Source: CAD feature listing. Evaluate the final solid. Frame: model axes, mm. A direction names the side the tool comes from. Round coordinates to 2 decimals unless told otherwise and drop trailing zeros. Write each loop counter-clockwise with the first axis right and the second up, starting at its lowest first coordinate (ties: lowest second). Pieces come first, ordered by that corner, then holes.
```python
from build123d import *

# Parameters (mm, degrees)
SKETCH1_W           = 15
SKETCH1_H           = 25.4
BOSS_EXTRUDE1_DEPTH = 3.175
SKETCH2_W           = 15
SKETCH2_H           = 3.175
BOSS_EXTRUDE2_DEPTH = 22.225
SKETCH3_R           = 1.5
CUT_EXTRUDE2_DEPTH  = 39.927111375
SKETCH4_R           = 1.5
CUT_EXTRUDE3_DEPTH  = 37.933868265


with BuildPart() as part:
    # Sketch1 → Boss-Extrude1 (new body)
    with BuildSketch(Plane(origin=(0, 0, 0), x_dir=(0, 0, -1), z_dir=(1, 0, 0))):
        with Locations((7.5, 12.7)):
            Rectangle(SKETCH1_W, SKETCH1_H)
    extrude(amount=BOSS_EXTRUDE1_DEPTH)

    # Sketch2 → Boss-Extrude2 (add)
    with BuildSketch(Plane(origin=(3.175, 0, 0), x_dir=(0, 0, -1), z_dir=(1, 0, 0))):
        with Locations((7.5, 1.5875)):
            Rectangle(SKETCH2_W, SKETCH2_H)
    extrude(amount=BOSS_EXTRUDE2_DEPTH)

    # Sketch3 → Cut-Extrude2 (cut, through all)
    with BuildSketch(Plane.XZ):
        with Locations(Location((7.5, -7.5, 0), (0, 0, 270))):
            Circle(SKETCH3_R)
        with Locations(Location((15, -7.5, 0), (0, 0, 270))):
            Circle(SKETCH3_R)
    extrude(amount=-CUT_EXTRUDE2_DEPTH, mode=Mode.SUBTRACT)

    # Sketch4 → Cut-Extrude3 (cut, through all)
    with BuildSketch(Plane(origin=(3.175, 0, 0), x_dir=(0, 0, -1), z_dir=(1, 0, 0))):
        with Locations((7.5, 17.9)):
            Circle(SKETCH4_R)
        with Locations((7.5, 10.4)):
            Circle(SKETCH4_R)
    extrude(amount=-CUT_EXTRUDE3_DEPTH, mode=Mode.SUBTRACT)


solid = part.part
```
Q1. Set-up query: faces 4 (the face through (2, 25.4, -7)), 5 (the face through (14, 3.175, -6)). Return all of +Z, -Z, +X, -X, +Y, -Y with unobstructed straight access to the full face (end or side cutting, diameter ignored); none if empty.
Q2. Mould query, pull axis X, two halves, no side actions, for faces 1 (the face through (0, 13, -7)), 2 (the face through (13, 0, -7)), 3 (the face through (6.036, 1.565, -7.175)). Classes: pulls with the +X half, pulls with the -X half, needs draft (parallel to the pull), parting line crosses it, or undercut.
Q3. Section query B-B, the plane x = 15. Output: boundary loops of the cut face in (y, z) (3 decimals).
Q4. Line query: line 1 (Y direction, x = 2.25, z = -7.5); line 2 (X direction, y = 1.15, z = -7.5); line 3 (X direction, y = 3.5, z = -7) (3 decimals). Output: solid intervals per line, ascending.
Q5. Pin query (flat end, axial travel): P1, Ø5, axis at x = 7.5, z = -7.5, coming from the +Y side (3 decimals); P2, Ø3, axis at y = 5.5, z = -2.5, coming from the +X side (3 decimals). Return the tip coordinate at first contact, or that it passes through.
Q6. Section query D-D, the plane y = 2. Output: boundary loops of the cut face in (x, z), and give its area (3 significant figures).
Q7. Section query A-A, the plane z = -7.5. Output: boundary loops of the cut face in (x, y) (3 decimals), and give its area (3 significant figures).
Filled in:
1. face 4: +Z, -Z, +X, -X, +Y
1. face 5: +Z, -Z, +X, +Y
2. face 1: pulls with the -X half
2. face 2: needs draft
2. face 3: undercut
3. outline: (0, -15) - (3.175, -15) - (3.175, -9) - (0, -9) - close; (0, -6) - (3.175, -6) - (3.175, 0) - (0, 0) - close
4. line 1: y = 0 to 8.9, 11.9 to 16.4, 19.4 to 25.4
4. line 2: x = 0 to 6, 9 to 13.5, 16.5 to 25.4
4. line 3: x = 0 to 3.175
5. P1: stops at y = 3.175
5. P2: stops at x = 3.175
6. outline: (0, -15) - (25.4, -15) - (25.4, 0) - (0, 0) - close; hole circle Ø3 at (7.5, -7.5); hole circle Ø3 at (15, -7.5)
6. area: 367 mm2
7. outline: (0, 0) - (6, 0) - (6, 3.175) - (3.175, 3.175) - (3.175, 8.9) - (0, 8.9) - close; (0, 11.9) - (3.175, 11.9) - (3.175, 16.4) - (0, 16.4) - close; (0, 19.4) - (3.175, 19.4) - (3.175, 25.4) - (0, 25.4) - close; (9, 0) - (13.5, 0) - (13.5, 3.175) - (9, 3.175) - close; (16.5, 0) - (25.4, 0) - (25.4, 3.175) - (16.5, 3.175) - close
7. area: 113 mm2
